Autodesk Inventor part; units mm, degrees
ref_plane "YZ Plane" through (0, 0, 0) normal (1, 0, 0) x (0, 1, 0)
ref_plane "XZ Plane" through (0, 0, 0) normal (0, 1, 0) x (-1, 0, 0)
ref_plane "XY Plane" through (0, 0, 0) normal (0, 0, 1) x (1, 0, 0)
sketch "Sketch1" plane through (0, 0, 0) normal (1, 0, 0) x (0, 1, 0)
  arc A0 (0.0036, 12) -> (0.0036, -12) centre (0.0036, 0) ccw
  circle A1 centre (0.0036, 0) radius 4.375
  circle A2 centre (0.0036, 0) radius 9 construction
  line L0 (-11.9964, 0) -> (0.0036, 0) construction
  line L1 (-8.9964, 0) -> (-7.7964, 0)
  circle A3 centre (-7.7964, 0) radius 1.2
  circle A4 centre (-3.8964, -6.755) radius 1.2
  circle A5 centre (3.9036, -6.755) radius 1.2
  circle A6 centre (7.8036, 0) radius 1.2
  circle A7 centre (3.9036, 6.755) radius 1.2
  circle A8 centre (-3.8964, 6.755) radius 1.2
  line L2 (-11.9964, 0) -> (33.0036, 0) construction
  line L3 (-11.9964, 37.6945) -> (46.0036, 37.6945) construction
  line L4 (0.0036, 12) -> (46.0036, 12)
  line L5 (46.0036, 12) -> (46.0036, -3)
  arc A9 (0.0036, -12) -> (7.4266, -9.4286) centre (0.0036, 0) ccw
  arc A10 (25.9843, -3) -> (7.4266, -9.4286) centre (25.9843, -33) ccw
  line L6 (25.9843, -3) -> (46.0036, -3)
  circle A11 centre (40.0036, 4.5) radius 1.5
  line L7 (31.5036, 6) -> (22.5036, 6)
  line L8 (22.5036, 6) -> (22.5036, 3)
  line L9 (22.5036, 3) -> (31.5036, 3)
  line L10 (31.5036, 3) -> (31.5036, 6)
  point P0 (1.5, 26.1095)
  point P1 (22.5, 26.1095)
  point P2 (-4.4964, -7.7942)
  point P3 (4.5036, -7.7942)
  point P4 (9.0036, 0)
  point P5 (4.5036, 7.7942)
  point P6 (-4.4964, 7.7942)
  point P7 (11.6225, -3)
  dimension "d4" = 18
  dimension "d2" = 24
  dimension "d3" = 8.75
  dimension "d5" = 1.2
  dimension "d7" = 360
  dimension "d8" = 45
  dimension "d12" = 12
  dimension "d15" = 58
  dimension "d16" = 15
  dimension "d18" = 30
  dimension "d22" = 3
  dimension "d23" = 6
  dimension "d28" = 7.5
  dimension "d29" = 15
  dimension "d31" = 9
  dimension "d32" = 3
  dimension "d33" = 12
extrude "Extrusion1" add sketch "Sketch1" along normal blind 3
properties part number "Brazo3"
Design review of the part built by this model. Coordinates are the model's own, in mm. A direction names the side the tool comes from. Give positions to 0.01 mm unless a question says otherwise; leave off trailing zeros. Loops run counter-clockwise (first coordinate to the right, second up) from the corner with the lowest first, then second, coordinate; pieces in that order, holes last. Notation, with made-up numbers: (-31, 52) -> (11, 52) arc R29 cw to (11, 72) -> close; hole circle Ø11 at (-25, 7.25). An arc over 180 degrees is marked (long way). One line per question, with ' | ' between items. Start each with the question number.
(1) We need section D-D (y = 16.5). State the section outline as (x, z) points, and give its area (3 significant figures).
(2) Insertion check: P1, Ø1.5, axis at x = 1.5, y = 25.5, coming from the -Z side; P2, Ø0.9, axis at x = 1.5, z = 5, coming from the -Y side. Each pin has a flat end and moves straight along its axis. Give the tip position at first contact, or say it passes through.
(3) We need section B-B (x = 0.9). State how many separate pieces and enclosed holes the cut face has, and give its area (3 significant figures).
(4) We need section C-C (y = 39.5). State the section outline as (x, z) points, and give its area (3 significant figures).
(5) We need section A-A (z = 0). State the section outline as (x, y) points, and give its area (3 significant figures).
(6) For faces 1 (the face through (0, 17, 3)), 2 (the face through (1, 36, -3)), 3 (the face through (1, 31.504, 4)), list the 3-axis set-ups (+Z, -Z, +X, -X, +Y, -Y) from which the entire face can be reached by the end or side of a thin tool; tool diameter is ignored.
(7) For line 1 (Z direction, x = 1.3, y = 27.5); line 2 (Z direction, x = 1.95, y = -4.5); line 3 (Y direction, x = 1.4, z = -7.5), list the stretches that pass through material, from the lowest coordinate up.
The answers:
1) outline: (0, -4.54) -> (3, -4.54) -> (3, 12) -> (0, 12) -> close | area: 49.6 mm^2
2) P1: stops at z = -3.03 | P2: stops at y = -11.1
3) separate pieces: 1 | enclosed holes: 9 | area: 893 mm^2
4) outline: (0, -3) -> (3, -3) -> (3, 3.09) -> (0, 3.09) -> close; (0, 5.91) -> (3, 5.91) -> (3, 12) -> (0, 12) -> close | area: 36.5 mm^2
5) outline: (0, -12) -> (3, -12) -> (3, -9) -> (0, -9) -> close; (0, -6.6) -> (3, -6.6) -> (3, -4.37) -> (0, -4.37) -> close; (0, 4.38) -> (3, 4.38) -> (3, 6.6) -> (0, 6.6) -> close; (0, 9) -> (3, 9) -> (3, 46) -> (0, 46) -> close | area: 133 mm^2
6) face 1: +Z, -Z, -X, +Y, -Y | face 2: -Z, +X, -X, +Y | face 3: +X, -X
7) line 1: z = -3 to 3, 6 to 12 | line 2: z = -11.12 to -7.79, -5.72 to 5.72, 7.79 to 11.12 | line 3: y = -9.36 to -4.84, -2.96 to 2.96, 4.84 to 10.18
